The model under review builds one solid part; all positions refer to its coordinate system, in mm. A direction names the side the tool comes from. Coordinates: 2 decimals unless noted, no trailing zeros. Order: outer loops, then holes, each group sorted by start corner. A loop starts at its lowest first (then second) coordinate and runs counter-clockwise, first axis right, second up.
Autodesk Inventor part; units mm, degrees
ref_plane "YZ Plane" through (0, 0, 0) normal (1, 0, 0) x (0, 1, 0)
ref_plane "XZ Plane" through (0, 0, 0) normal (0, 1, 0) x (-1, 0, 0)
ref_plane "XY Plane" through (0, 0, 0) normal (0, 0, 1) x (1, 0, 0)
sketch "Sketch1" plane through (0, 0, 0) normal (0, 0, 1) x (1, 0, 0)
  line L0 (12.5, -112.2169) -> (-12.5, -112.2169)
  line L1 (-12.5, -112.2169) -> (-12.5, 112.2169)
  line L2 (-12.5, 112.2169) -> (12.5, 112.2169)
  line L3 (12.5, 112.2169) -> (12.5, -112.2169)
  line L4 (12.5, -112.2169) -> (-12.5, 112.2169) construction
  line L5 (-12.5, -112.2169) -> (12.5, 112.2169) construction
  line L6 (0, 105) -> (0, -105) construction
  line L7 (-12.5, 112.2169) -> (0, 119.4338)
  line L8 (0, 119.4338) -> (12.5, 112.2169)
  line L9 (12.5, 112.2169) -> (12.5, 97.7831)
  line L10 (12.5, 97.7831) -> (0, 90.5662)
  line L11 (0, 90.5662) -> (-12.5, 97.7831)
  line L12 (-12.5, 97.7831) -> (-12.5, 112.2169)
  line L13 (-12.5, -112.2169) -> (-12.5, -97.7831)
  line L14 (-12.5, -97.7831) -> (0, -90.5662)
  line L15 (0, -90.5662) -> (12.5, -97.7831)
  line L16 (12.5, -97.7831) -> (12.5, -112.2169)
  line L17 (12.5, -112.2169) -> (0, -119.4338)
  line L18 (0, -119.4338) -> (-12.5, -112.2169)
  line L19 (-4.1551, 106.7278) -> (4.1551, 103.2722) construction
  line L20 (-4.9806, 104.7427) -> (3.3295, 101.287)
  line L21 (4.9806, 105.2573) -> (-3.3295, 108.713)
  arc A0 (-3.3295, 108.713) -> (-4.9806, 104.7427) centre (-4.1551, 106.7278) ccw
  arc A1 (3.3295, 101.287) -> (4.9806, 105.2573) centre (4.1551, 103.2722) ccw
  circle A2 centre (0, -105) radius 3.5
  line L22 (18.5, -67.75) -> (-18.5, -67.75)
  line L23 (-18.5, -67.75) -> (-18.5, 67.75)
  line L24 (-18.5, 67.75) -> (18.5, 67.75)
  line L25 (18.5, 67.75) -> (18.5, -67.75)
  line L26 (18.5, -67.75) -> (-18.5, 67.75) construction
  line L27 (-18.5, -67.75) -> (18.5, 67.75) construction
  circle A3 centre (0, 0) radius 12.7
  point P0 (252.5, 0)
  point P1 (-12.5, -67.75)
  point P2 (12.5, -112.2169)
  point P3 (-12.5, 67.75)
  point P4 (12.5, 67.75)
  point P5 (12.5, -67.75)
  point P6 (12.5, 97.7831)
  point P7 (-12.5, 112.2169)
  point P8 (12.5, -97.7831)
  point P9 (-12.5, -112.2169)
  point P10 (12.5, -112.2169)
  point P11 (12.5, -2.245)
  point P12 (-12.5, -2.245)
  point P13 (-12.5, 2.245)
  point P14 (12.5, 2.245)
  dimension "d0" = 25
  dimension "d1" = 252.5
  dimension "d2" = 210
  dimension "d3" = 4.3
  dimension "d4" = 9
  dimension "d5" = 7
  dimension "d12" = 135.5
  dimension "d13" = 37
  dimension "d43" = 25.4
extrude "Extrusion1" add sketch "Sketch1" along normal blind 6.35
sketch "Sketch2" plane through (0, 0, 6.35) normal (0, 0, 1) x (1, 0, 0)
  line L0 (-18.5, 67.75) -> (-18.5, -67.75)
  line L1 (-18.5, -67.75) -> (-12.5, -67.75)
  line L2 (-12.5, -67.75) -> (-12.5, -112.2169)
  line L3 (-12.5, -112.2169) -> (0, -119.4338)
  line L4 (0, -119.4338) -> (12.5, -112.2169)
  line L5 (12.5, -112.2169) -> (12.5, -67.75)
  line L6 (12.5, -67.75) -> (18.5, -67.75)
  line L7 (18.5, -67.75) -> (18.5, 67.75)
  line L8 (18.5, 67.75) -> (12.5, 67.75)
  line L9 (12.5, 67.75) -> (12.5, 112.2169)
  line L10 (12.5, 112.2169) -> (0, 119.4338)
  line L11 (0, 119.4338) -> (-12.5, 112.2169)
  line L12 (-12.5, 112.2169) -> (-12.5, 67.75)
  line L13 (-12.5, 67.75) -> (-18.5, 67.75)
  arc A0 (-3.3295, 108.713) -> (-4.9806, 104.7427) centre (-4.1551, 106.7278) ccw
  line L14 (-3.3295, 108.713) -> (4.9806, 105.2573)
  arc A1 (3.3295, 101.287) -> (4.9806, 105.2573) centre (4.1551, 103.2722) ccw
  line L15 (3.3295, 101.287) -> (-4.9806, 104.7427)
  circle A2 centre (0, -105) radius 3.5
  circle A3 centre (-13.25, 68.5) radius 1.375
  point P0 (0, 0)
  point P1 (-12.5, 69.6524)
  point P2 (-14.4024, 67.75)
  dimension "d16" = 0.75
  dimension "d17" = 2.75
  dimension "d18" = 0.75
extrude "Extrusion2" cut sketch "Sketch2" against normal through all contours L13 L12 A3 picked at (-12.4132, 68.945)
mirror "Mirror1" about plane through (0, 0, 0) normal (1, 0, 0) of "Extrusion2"
mirror "Mirror2" about plane through (0, 0, 0) normal (0, 1, 0) of "Extrusion2", "Mirror1"
sketch "Sketch4" plane through (0, 0, 6.35) normal (0, 0, 1) x (1, 0, 0)
  line L0 (-18.5, -67.75) -> (-14.4024, -67.75) construction
  line L1 (10, -58) -> (-10, -58) construction
  line L2 (-10, -58) -> (-10, 58) construction
  line L3 (-10, 58) -> (10, 58) construction
  line L4 (10, 58) -> (10, -58) construction
  line L5 (10, -58) -> (-10, 58) construction
  line L6 (-10, -58) -> (10, 58) construction
  point P0 (0, 0)
  point P1 (10, 0)
  point P2 (-10, 0)
  dimension "d45" = 20
  dimension "d46" = 116
hole "Hole2" at (10, -58, 6.35) at (-10, -58, 6.35) at (-10, 0, 6.35) at (10, 0, 6.35) at (10, 58, 6.35) at (-10, 58, 6.35) direction (0, 0, -1) diameter 5.3 end through all
fillet "Fillet3" radius 1 18 edges at (-18.5, 67.75, 3.175) (-18.5, -67.75, 3.175) (14.4024, -67.75, 3.175) (-14.4024, -67.75, 3.175) (-12.5, -69.6524, 3.175) (18.5, -67.75, 3.175) (12.5, -69.6524, 3.175) (0, -119.4338, 3.175) (12.5, -112.2169, 3.175) (-12.5, -112.2169, 3.175) (18.5, 67.75, 3.175) (-14.4024, 67.75, 3.175) (14.4024, 67.75, 3.175) (0, 119.4338, 3.175) (-12.5, 112.2169, 3.175) (-12.5, 69.6524, 3.175) (12.5, 69.6524, 3.175) (12.5, 112.2169, 3.175)
equation "\"d18\" = d16"
properties part number "Z-Axis Nut and Bed Plate RevIII" material "Aluminum 6061"
(1) We need section B-B, the plane z = 2.25. Count the separate pieces of the cut face and the enclosed holes in it, and give its area (3 significant figures).
A:
separate pieces: 1
enclosed holes: 8
area: 7,180 mm2
(2) Wall thickness on probe 1 along X at (y, z) = (0.5, 3.75); probe 2 along Y at (x, z) = (10, 1.75); probe 3 along Y at (x, z) = (-1, 2.5): over which ranges is each line inside the solid? List them lowest first.
A:
probe 1: x = -18.5 to -12.6, -7.4 to 7.4, 12.6 to 18.5
probe 2: y = -113.66 to -60.65, -55.35 to -2.65, 2.65 to 55.35, 60.65 to 113.66
probe 3: y = -118.86 to -108.35, -101.65 to 103.09, 107.74 to 118.86
(3) Machinability: for faces 1 (the face through (0.884, 106.961, 3.131)), 2 (the face through (12.5, -91, 3)), 3 (the face through (-12.5, 91, 3)), which of the approach directions +Z, -Z, +X, -X, +Y, -Y give a long, thin tool a straight path to every point of the face, cutting with its end or side? Answer none if there is none.
A:
face 1: +Z, -Z
face 2: +Z, -Z, +X, -Y
face 3: +Z, -Z, -X, +Y
(4) We need section C-C, the plane y = 79. Write out the cut boundary in (x, z), and give its area (3 significant figures).
A:
outline: (-12.5, 0) - (12.5, 0) - (12.5, 6.35) - (-12.5, 6.35) - close
area: 159 mm2
(5) We need section A-A, the plane y = 0. Write out the cut boundary in (x, z), and give its area (3 significant figures).
A:
outline: (-18.5, 0) - (-12.65, 0) - (-12.65, 6.35) - (-18.5, 6.35) - close; (-7.35, 0) - (7.35, 0) - (7.35, 6.35) - (-7.35, 6.35) - close; (12.65, 0) - (18.5, 0) - (18.5, 6.35) - (12.65, 6.35) - close
area: 168 mm2
(6) For pin 1 Ø0.8 at (x, z) = (-16.5, 1.5) entering from +Y; pin 2 Ø3 at (y, z) = (93, 4) entering from -X; pin 3 Ø1.3 at (x, z) = (15.5, 2.5) entering from -Y, all flat-tipped, find the tip position at first contact; note any pin that passes through.
A:
pin 1: stops at y = 67.75
pin 2: stops at x = -12.5
pin 3: stops at y = -67.75
(7) Draft analysis for pull direction X (two halves, no side actions). For faces 4 (the face through (-8.99, 55.55, 3.13)), 5 (the face through (6.33, -115.78, 3.13)), 6 (the face through (-0.884, 103.039, 3.131)), 7 (the face through (-12.5, -91, 3)), state which applies: released by +X, released by -X, zero draft, split by the parting line, or undercut.
A:
face 4: undercut
face 5: released by +X
face 6: undercut
face 7: released by -X
